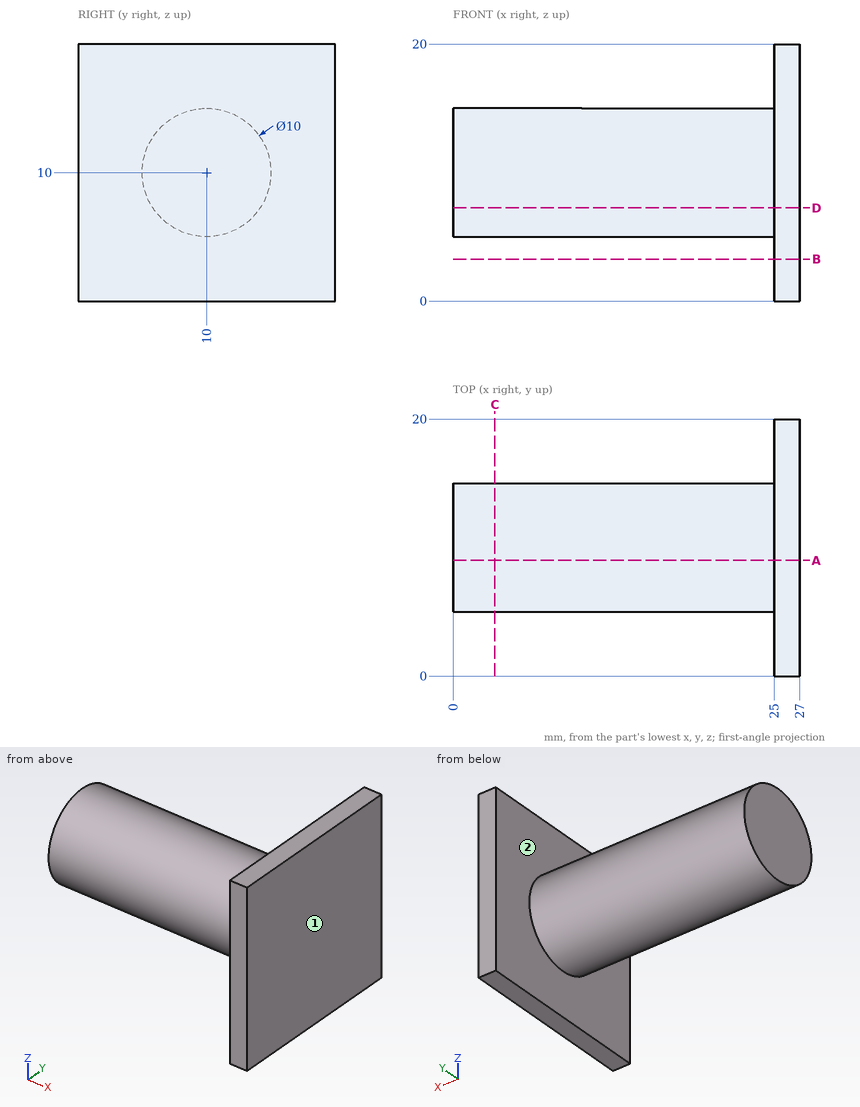
Answer from the drawing. Dimensions are ordinates in mm from the lowest x, y and z of the part. A direction names the side the tool comes from. Give positions to 0.01 mm unless a question says otherwise; leave off trailing zeros. Write each loop counter-clockwise with the first axis right and the second up, starting at its lowest first coordinate (ties: lowest second). Pieces come first, ordered by that corner, then holes.
1) Given P1, Ø4, axis at x = 22.5, y = 8.5, coming from the -Z side; P2, Ø1.5, axis at y = 3.5, z = 16.5, coming from the -X side; P3, Ø10, axis at x = 6, z = 13, coming from the +Y side, each flat-ended and moving along its own axis, determine where each tip first touches the part or whether it passes through.
2) Find the intervals of material crossed by L1, parallel to X at y = 1.5, z = 18; L2, parallel to Y at x = 16, z = 10; L3, parallel to Y at x = 21, z = 7.5, in increasing order.
3) Section C-C (x = 3.25) is taken. Write down the section's boundary in (y, z), and give its area (3 significant figures).
4) Section B-B (z = 3.25) is taken. Write down the section's boundary in (x, y), and give its area (3 significant figures).
5) Section A-A (y = 9) is taken. Write down the section's boundary in (x, z).
6) A tool of negligible diameter and unlimited length cuts with its end or side. For the marked faces 1 and 2, from which of +Z, -Z, +X, -X, +Y, -Y can it reach the whole face along a straight path? Write none if from no direction.
7) Section D-D (z = 7.25) is taken. Write down the section's boundary in (x, y).
Response:
1. P1: stops at z = 5
1. P2: stops at x = 25
1. P3: stops at y = 15
2. L1: x = 25 to 27
2. L2: y = 5 to 15
2. L3: y = 5.67 to 14.33
3. outline: circle Ø10 at (10, 10)
3. area: 78.5 mm2
4. outline: (25, 0) - (27, 0) - (27, 20) - (25, 20) - close
4. area: 40.0 mm2
5. outline: (0, 5.1) - (25, 5.1) - (25, 0) - (27, 0) - (27, 20) - (25, 20) - (25, 14.9) - (0, 14.9) - close
6. face 1: +Z, -Z, +X, +Y, -Y
6. face 2: -X
7. outline: (0, 5.82) - (25, 5.82) - (25, 0) - (27, 0) - (27, 20) - (25, 20) - (25, 14.18) - (0, 14.18) - close
